Study the drawing (mm; zero at the part's minimum x, y, z) and answer. A direction names the side the tool comes from. Round coordinates to 2 decimals unless told otherwise and drop trailing zeros. Order: outer loops, then holes, each group sorted by start corner. A loop starts at its lowest first (then second) coordinate and runs counter-clockwise, first axis right, second up. Notation, with made-up numbers: (57, -12) -> (74, -12) arc R8 ccw to (74, -1) -> close; hole circle Ø2 at (48, 13.25). An arc over 180 degrees is marked (long way). Use one line per item in the form item = value.
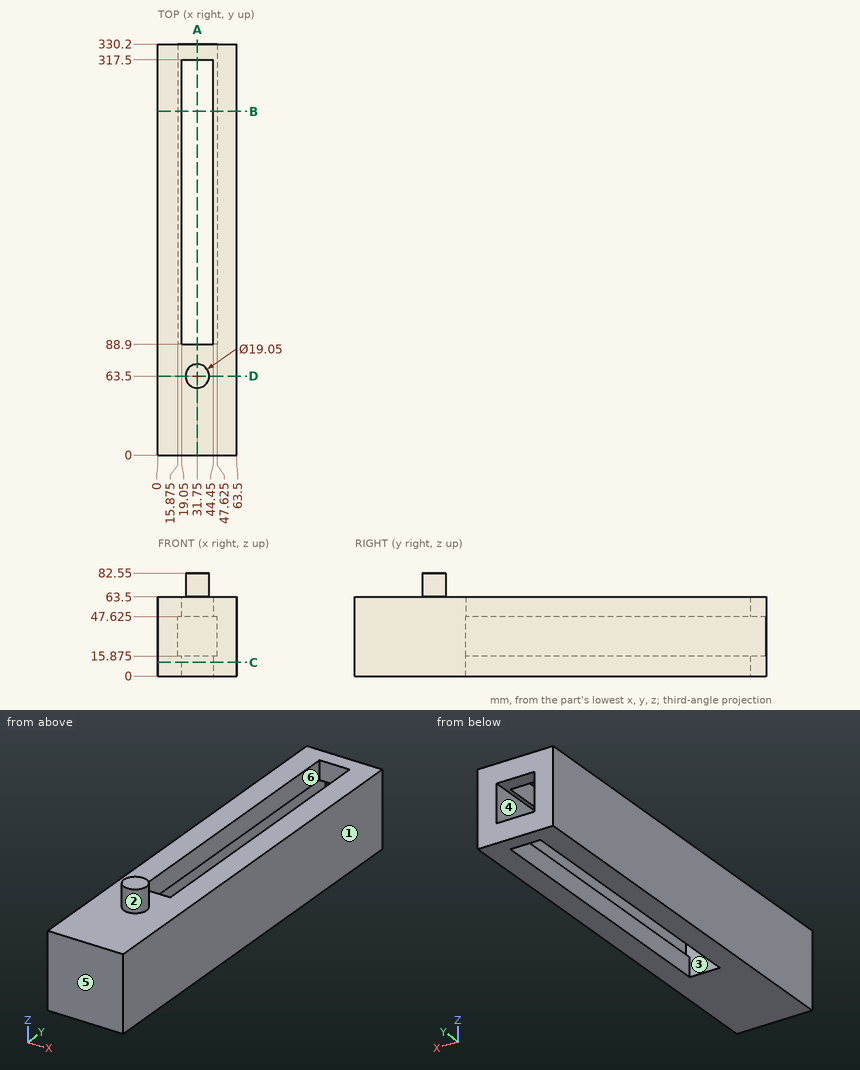
Item 1: Consider line 1 along X through (y, z) = (144, 23) (3 decimals); line 2 along X through (y, z) = (121.5, 60.5). Determine where each line is inside the solid, lowest interval first.
Findings:
line_1 = 0 to 15.875, 47.625 to 63.5
line_2 = 0 to 19.05, 44.45 to 63.5
Item 2: For the marked faces 4, 5 and 6, determine the directions among +Z, -Z, +X, -X, +Y, -Y from which every point of the face is accessible in a straight line to the end or side of a thin tool.
Findings:
face_4 = +Y
face_5 = +Z, -Z, +X, -X, -Y
face_6 = +Z, -Z
Item 3: Flat-ended cylindrical pins translate along their axes: P1, Ø9.5, axis at x = 37, y = 157, coming from the +Z side; P2, Ø16, axis at x = 26.5, z = 30, coming from the +Y side; P3, Ø2, axis at x = 14, y = 141.5, coming from the +Z side. Find the tip coordinate at first contact, or state that the pin passes through.
Findings:
P1 = through
P2 = 88.9
P3 = 63.5
Item 4: The part is cut by section C-C, the plane z = 11. Give the vertices of the cut face in (x, y).
Findings:
outline = (0, 0) -> (63.5, 0) -> (63.5, 330.2) -> (0, 330.2) -> close; hole (19.05, 88.9) -> (44.45, 88.9) -> (44.45, 317.5) -> (19.05, 317.5) -> close
Item 5: The part is cut by section B-B, the plane y = 276. Give the vertices of the cut face in (x, z) (3 decimals), and give its area (3 significant figures).
Findings:
outline = (0, 0) -> (19.05, 0) -> (19.05, 15.875) -> (15.875, 15.875) -> (15.875, 47.625) -> (19.05, 47.625) -> (19.05, 63.5) -> (0, 63.5) -> close; (44.45, 0) -> (63.5, 0) -> (63.5, 63.5) -> (44.45, 63.5) -> (44.45, 47.625) -> (47.625, 47.625) -> (47.625, 15.875) -> (44.45, 15.875) -> close
area = 2,220 mm^2
Item 6: The part is cut by section D-D, the plane y = 63.5. Give the vertices of the cut face in (x, z) (3 decimals).
Findings:
outline = (0, 0) -> (63.5, 0) -> (63.5, 63.5) -> (41.275, 63.5) -> (41.275, 82.55) -> (22.225, 82.55) -> (22.225, 63.5) -> (0, 63.5) -> close
Item 7: Determine the mould class of the marked faces 1, 2 and 3 for opening direction Y: released by +Y, released by -Y, zero draft, split by the parting line, or undercut.
Findings:
face_1 = zero draft
face_2 = split by the parting line
face_3 = undercut
Item 8: The part is cut by section A-A, the plane x = 31.75. Give the vertices of the cut face in (y, z) (3 decimals), and give its area (3 significant figures).
Findings:
outline = (0, 0) -> (88.9, 0) -> (88.9, 63.5) -> (73.025, 63.5) -> (73.025, 82.55) -> (53.975, 82.55) -> (53.975, 63.5) -> (0, 63.5) -> close; (317.5, 0) -> (330.2, 0) -> (330.2, 15.875) -> (317.5, 15.875) -> close; (317.5, 47.625) -> (330.2, 47.625) -> (330.2, 63.5) -> (317.5, 63.5) -> close
area = 6,410 mm^2
